Answer from the drawing. Dimensions are ordinates in mm from the lowest x, y and z of the part. A direction names the side the tool comes from. Give positions to 0.01 mm unless a question says otherwise; leave off trailing zeros. Write each loop counter-clockwise with the first axis right and the second up, starting at its lowest first coordinate (ties: lowest second). Pieces come first, ordered by that corner, then holes. Notation, with made-up numbers: (14, 64) -> (47, 64) arc R21 ccw to (47, 89) -> close; hole circle Ø6 at (-33, -7.5). An arc over 180 degrees is marked (long way). Use a Markdown table: item, result. Add a question column.
Q1. For the marked faces 4, 5 and 6, determine the directions among +Z, -Z, +X, -X, +Y, -Y from which every point of the face is accessible in a straight line to the end or side of a thin tool.
Q2. Each of these flat-tipped pins is pushed along its axis until it touches: pin 1 Ø2.5 at (x, z) = (13.5, 19) entering from +Y; pin 2 Ø1.5 at (x, z) = (13.5, 7) entering from -Y; pin 3 Ø2 at (x, y) = (2, 17.5) entering from +Z. Where does it stop, or does it pass through?
Q3. Section B-B, the plane z = 12.5 is taken. Give the vertices of the cut face in (x, y) (1 decimal), plus the area to 3 significant figures.
Q4. Section C-C, the plane x = 13.5 is taken. State how many separate pieces and enclosed holes the cut face has.
Q5. Section D-D, the plane x = 2 is taken. Give the vertices of the cut face in (y, z), plus the area to 3 significant figures.
Q6. Section A-A, the plane y = 12.5 is taken. Give the vertices of the cut face in (x, z) (1 decimal).
Q7. Consider line 1 (X direction, y = 10.5, z = 5.5); line 2 (Z direction, x = 13.5, y = 10.85) (1 decimal); line 3 (Z direction, x = 13.5, y = 10.4). Determine where each line is inside the solid, lowest interval first.
Q8. For a pull along Z with two mould halves and no side action, classify the marked faces 1, 2 and 3 as pulls with the +Z half, pulls with the -Z half, needs draft (parallel to the pull), parting line crosses it, or undercut.
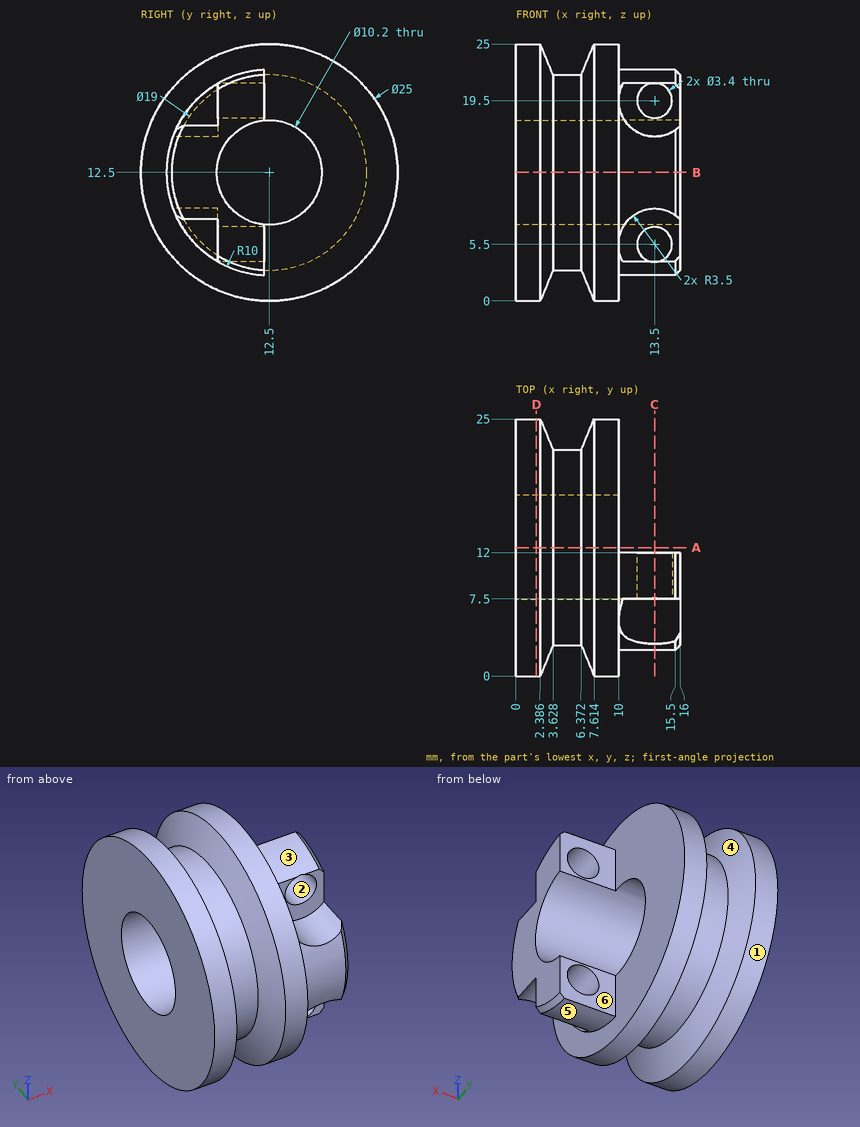
Result set:
| question | item | result |
|---|---|---|
| 1 | face 4 | none |
| 1 | face 5 | -Z, +X, -Y |
| 1 | face 6 | +Z, -Z, +X, +Y |
| 2 | pin 1 | stops at y = 12 |
| 2 | pin 2 | stops at y = 7.5 |
| 2 | pin 3 | stops at z = 24.34 |
| 3 | outline | (0, 0) -> (2.4, 0) -> (3.6, 3) -> (6.4, 3) -> (7.6, 0) -> (10, 0) -> (10, 2.5) -> (15.5, 2.5) -> (16, 3) -> (16, 7.4) -> (0, 7.4) -> close; (0, 17.6) -> (10, 17.6) -> (10, 25) -> (7.6, 25) -> (6.4, 22) -> (3.6, 22) -> (2.4, 25) -> (0, 25) -> close |
| 3 | area | 153 mm2 |
| 4 | separate pieces | 3 |
| 4 | enclosed holes | 0 |
| 5 | outline | circle Ø25 at (12.5, 12.5); hole circle Ø10.2 at (12.5, 12.5) |
| 5 | area | 409 mm2 |
| 6 | outline | (0, 0) -> (2.4, 0) -> (3.6, 3) -> (6.4, 3) -> (7.6, 0) -> (10, 0) -> (10, 7.4) -> (0, 7.4) -> close; (0, 17.6) -> (10, 17.6) -> (10, 25) -> (7.6, 25) -> (6.4, 22) -> (3.6, 22) -> (2.4, 25) -> (0, 25) -> close |
| 7 | line 1 | x = 0 to 11.8, 15.2 to 16 |
| 7 | line 2 | z = 2.6 to 3.8, 7.2 to 7.7, 17.3 to 17.8, 21.2 to 22.4 |
| 7 | line 3 | z = 2.72 to 3.8, 7.2 to 7.85, 17.15 to 17.8, 21.2 to 22.28 |
| 8 | face 1 | parting line crosses it |
| 8 | face 2 | undercut |
| 8 | face 3 | pulls with the +Z half |
